Input: part model. Units: mm. Frame: model coordinates. A direction names the side the tool comes from. Give positions to 0.01 mm unless a question says otherwise; leave off trailing zeros. Loops run counter-clockwise (first coordinate to the right, second up) from the corner with the lowest first, then second, coordinate; pieces in that order, holes last. Notation, with made-up numbers: (82, -12) -> (127, -12) arc R19 ccw to (127, 22) -> close; hole circle Ø3 at (31, 21.25). An arc over 180 degrees is marked (long way). One line per question, with ' | ' between items.
from build123d import *

# Parameters (mm, degrees)
BOSS_EXTRUDE1_DEPTH = 20
SKETCH2_R           = 1.775
CUT_EXTRUDE1_DEPTH  = 5
FILLET1_R           = 3
FILLET2_R           = 5


with BuildPart() as part:
    # Sketch1 → Boss-Extrude1 (new body)
    with BuildSketch(Plane(origin=(0, 0, 0), x_dir=(1, 0, 0), z_dir=(0, 1, 0))):
        with BuildLine():
            Line((0, 0), (0, 4))
            Line((0, 4), (24, 4))
            Line((24, 4), (24, 12))
            ThreePointArc((24, 12), (42, 30), (60, 12))
            Line((60, 12), (60, 4))
            Line((60, 4), (84, 4))
            Line((84, 4), (84, 0))
            Line((84, 0), (54.7, 0))
            Line((54.7, 0), (54.7, 12))
            ThreePointArc((54.7, 12), (42, 24.7), (29.3, 12))
            Line((29.3, 12), (29.3, 0))
            Line((29.3, 0), (0, 0))
        make_face()
    extrude(amount=BOSS_EXTRUDE1_DEPTH)

    # Sketch2 → Cut-Extrude1 (cut, through all)
    with BuildSketch(Plane(origin=(0, 0, -4), x_dir=(-1, 0, 0), z_dir=(0, 0, -1))):
        with Locations((-72, 10)):
            Circle(SKETCH2_R)
        with Locations((-12, 10)):
            Circle(SKETCH2_R)
    extrude(amount=-CUT_EXTRUDE1_DEPTH, mode=Mode.SUBTRACT)

    # Fillet1
    fillet1_edges = [part.edges().sort_by_distance(p)[0] for p in [
        (0, 0, -2),
        (84, 0, -2),
        (84, 20, -2),
        (0, 20, -2),
    ]]
    fillet(fillet1_edges, radius=FILLET1_R)

    # Fillet2
    fillet2_edges = [part.edges().sort_by_distance(p)[0] for p in [
        (24, 10, -4),
        (60, 10, -4),
    ]]
    fillet(fillet2_edges, radius=FILLET2_R)


solid = part.part
1. Section query A-A (y = 10). Output: boundary loops of the cut face in (x, z) (3 decimals).
Determined:
outline: (0, -4) -> (10.225, -4) -> (10.225, 0) -> (0, 0) -> close; (13.775, -4) -> (19, -4) arc R5 cw to (24, -9) -> (24, -12) arc R18 ccw to (60, -12) -> (60, -9) arc R5 cw to (65, -4) -> (70.225, -4) -> (70.225, 0) -> (54.7, 0) -> (54.7, -12) arc R12.7 cw to (29.3, -12) -> (29.3, 0) -> (13.775, 0) -> close; (73.775, -4) -> (84, -4) -> (84, 0) -> (73.775, 0) -> close
2. Section query C-C (x = 72). Output: boundary loops of the cut face in (y, z) (3 decimals), then the cut area to 3 significant figures.
Determined:
outline: (0, -4) -> (8.225, -4) -> (8.225, 0) -> (0, 0) -> close; (11.775, -4) -> (20, -4) -> (20, 0) -> (11.775, 0) -> close | area: 65.8 mm2
3. Pin query (flat end, axial travel): P1, Ø2.5, axis at y = 6, z = -10.5, coming from the -X side; P2, Ø4.5, axis at x = 12, y = 10, coming from the -Z side; P3, Ø4, axis at y = 13.5, z = -21, coming from the +X side. Return the tip coordinate at first contact, or that it passes through.
Determined:
P1: stops at x = 24 | P2: stops at z = -4 | P3: stops at x = 58.58
4. Ray query, line 1 along X through (y, z) = (6.75, -23.5); line 2 along X through (y, z) = (11.5, -10); line 3 along Z through (x, y) = (65.5, 5). Return the intervals inside material, ascending. Write a range as from..to.
Determined:
line 1: x = 28.15..36.61, 47.39..55.85 | line 2: x = 24..29.3, 54.7..60 | line 3: z = -4..0
5. Section query B-B (z = -3). Output: boundary loops of the cut face in (x, y) (3 decimals), then the cut area to 3 significant figures.
Determined:
outline: (0, 3) arc R3 ccw to (3, 0) -> (29.3, 0) -> (29.3, 20) -> (3, 20) arc R3 ccw to (0, 17) -> close; (54.7, 0) -> (81, 0) arc R3 ccw to (84, 3) -> (84, 17) arc R3 ccw to (81, 20) -> (54.7, 20) -> close; hole circle Ø3.55 at (12, 10); hole circle Ø3.55 at (72, 10) | area: 1,140 mm2
6. Reachability of faces 1 (the flat face through (60, 10, -11)), 2 (the flat face through (29.3, 10, -6)), 3 (the flat face through (54, 0, -17)), 4 (the flat face through (9, 10, -4)) from +Z, -Z, +X, -X, +Y, -Y: full face, straight path, thin tool, end or side. Return the list, or none.
Determined:
face 1: -Z, +X, +Y, -Y | face 2: +Z, +Y, -Y | face 3: +Z, -Z, +X, -X, -Y | face 4: -Z, -X, +Y, -Y
7. Pull-direction query (X, two-part tool) for faces 5 (the flat face through (54, 20, -17)), 6 (the flat face through (54.7, 10, -6)), 7 (the flat face through (24, 10, -10)); classes: pulls with the +X half, pulls with the -X half, needs draft (parallel to the pull), parting line crosses it, or undercut.
Determined:
face 5: needs draft | face 6: undercut | face 7: pulls with the -X half
8. Section query D-D (z = -15.5). Output: boundary loops of the cut face in (x, y).
Determined:
outline: (24.34, 0) -> (29.79, 0) -> (29.79, 20) -> (24.34, 20) -> close; (54.21, 0) -> (59.66, 0) -> (59.66, 20) -> (54.21, 20) -> close
